Autodesk Inventor part; units mm, degrees
ref_plane "YZ Plane" through (0, 0, 0) normal (1, 0, 0) x (0, 1, 0)
ref_plane "XZ Plane" through (0, 0, 0) normal (0, 1, 0) x (-1, 0, 0)
ref_plane "XY Plane" through (0, 0, 0) normal (0, 0, 1) x (1, 0, 0)
sketch "Sketch1" plane through (0, 0, 0) normal (0, 1, 0) x (-1, 0, 0)
  circle A0 centre (0, 0) radius 15.875
  dimension "d0" = 31.75
extrude "Extrusion1" add sketch "Sketch1" along normal blind 2.4892
sketch "Sketch2" plane through (0, 2.4892, 0) normal (0, 1, 0) x (1, 0, 0)
  circle A0 centre (0, 0) radius 15.875
  circle A1 centre (0, 11.5062) radius 1.8542
  line L0 (0, 0) -> (0, 15.875)
  circle A2 centre (-9.9647, -5.7531) radius 1.8542
  circle A3 centre (9.9647, -5.7531) radius 1.8542
  circle A4 centre (0, -25.4) radius 15.875
  line L1 (0, 0) -> (0, -25.4)
  circle A5 centre (21.997, 12.7) radius 15.875
  circle A6 centre (-21.997, 12.7) radius 15.875
  dimension "d3" = 3.7084
  dimension "d4" = 11.5062
  dimension "d7" = 360
  dimension "d9" = 31.75
  dimension "d10" = 25.4
  dimension "d13" = 360
extrude "Extrusion2" cut sketch "Sketch2" against normal through all contours A0 A5 | A0 A5 | A4 A0 | A0 L1 A4 | A6 A0 | A0 A6 | A0 A4 L1
sketch "Sketch6" plane through (0, 2.4892, 0) normal (0, 1, 0) x (1, 0, 0)
  arc A0 (-15.761, -1.8989) -> (-9.525, -12.7) centre (0, 0) ccw
  arc A1 (6.236, 14.5989) -> (-6.236, 14.5989) centre (0, 0) ccw
  line L0 (0, 0) -> (0, 11.5062)
  circle A2 centre (0, 11.5062) radius 1.8542
  circle A3 centre (-9.9647, -5.7531) radius 1.8542
  circle A4 centre (9.9647, -5.7531) radius 1.8542
  arc A5 (9.525, -12.7) -> (15.761, -1.8989) centre (0, 0) ccw
  circle A6 centre (0, 0) radius 4.5
  dimension "d26" = 11.5062
  dimension "d27" = 3.7084
  dimension "d30" = 360
  dimension "d34" = 9
extrude "Extrusion5" cut sketch "Sketch6" against normal through all
sketch "Sketch3" plane through (0, 2.4892, 0) normal (0, 1, 0) x (1, 0, 0)
  arc A0 (9.525, -12.7) -> (15.761, -1.8989) centre (0, 0) ccw
  circle A1 centre (0, 0) radius 5.9944
  line L0 (0, -7.3323) -> (-6.35, 3.6662)
  line L1 (-6.35, 3.6662) -> (6.35, 3.6662)
  line L2 (6.35, 3.6662) -> (0, -7.3323)
  line L3 (0, 0) -> (0, -8.4562)
  dimension "d17" = 11.9888
  dimension "d18" = 12.7
extrude "Extrusion3" add sketch "Sketch3" along normal blind 10.0076
sketch "Sketch4" plane through (0, 12.4968, 0) normal (0, 1, 0) x (1, 0, 0)
  arc A0 (-5.5463, 2.2741) -> (-0.8037, -5.9403) centre (0, 0) ccw
  circle A1 centre (0, 0) radius 3.9687
  dimension "d21" = 7.9375
extrude "Extrusion4" cut sketch "Sketch4" against normal through all
thread "Thread1"
properties part number "5_16_18_tee_nut"
Verification items for the finished model (mm, model axes). A direction names the side the tool comes from. Round coordinates to 2 decimals unless told otherwise and drop trailing zeros. Order: outer loops, then holes, each group sorted by start corner. A loop starts at its lowest first (then second) coordinate and runs counter-clockwise, first axis right, second up.
1. Section check D-D on z = 3.25. Record the cut outline in (x, y).
Final values:
outline: (-15.54, 0) - (-3.11, 0) - (-3.11, 2.49) - (-2.28, 2.49) - (-2.28, 12.5) - (-5.04, 12.5) - (-5.04, 2.49) - (-15.54, 2.49) - close; (2.28, 2.49) - (3.11, 2.49) - (3.11, 0) - (15.54, 0) - (15.54, 2.49) - (5.04, 2.49) - (5.04, 12.5) - (2.28, 12.5) - close
2. Section check B-B on x = -10. Record the cut outline in (y, z), then the cut area to 3 significant figures.
Final values:
outline: (0, -2.3) - (2.49, -2.3) - (2.49, 3.9) - (0, 3.9) - close; (0, 7.61) - (2.49, 7.61) - (2.49, 12.33) - (0, 12.33) - close
area: 27.2 mm2
3. Go/stop test with flat-tipped pins: P1, Ø1.8, axis at x = 6, y = 7.5, coming from the -Z side; P2, Ø1.5, axis at x = 12.5, y = 1.5, coming from the +Z side; P3, Ø3, axis at y = 7, z = -0.5, coming from the +X side. Record where each tip stops, or that it passes through.
Final values:
P1: stops at z = -3.67
P2: stops at z = 10.67
P3: stops at x = 5.99
4. Access from +Z, -Z, +X, -X, +Y, -Y to the whole of each face (thin tool, end or side, straight path). Record for faces 5 (the flat face through (5.954, 7.423, -2.98)), 6 (the flat face through (-6, 7, -3.666)), 7 (the flat face through (6, 7, -3.666)), 8 (the cylindrical face through (-0.59, 1.26, -4.46)), 9 (the flat face through (-0.396, 7.423, 6.646)).
Final values:
face 5: +X, +Y
face 6: -Z, -X, +Y
face 7: -Z, +X, +Y
face 8: -Y
face 9: +Z, -X, +Y
5. Thickness scan on L1, parallel to Z at x = 0, y = 1.45 (3 decimals); L2, parallel to X at y = 5.25, z = 0; L3, parallel to Z at x = -0.5, y = 7. Record the ranges inside material, lowest first.
Final values:
L1: z = -15.875 to -13.36, -9.652 to -4.5, 4.5 to 9.525
L2: x = -5.99 to -3.97, 3.97 to 5.99
L3: z = -5.97 to -3.94, 3.94 to 6.47
6. Release check for a two-part mould opening along X. For faces 1 (the cylindrical face through (5.23, 7.42, 2.93)), 2 (the flat face through (0, 0, -5)), 3 (the cylindrical face through (-0.077, 7.423, -5.994)), 4 (the cylindrical face through (0.143, 1.262, 9.526)) record: +X half, -X half, draft (parallel to the pull), parting line (faces both ways), or undercut.
Final values:
face 1: +X half
face 2: draft
face 3: parting line
face 4: undercut
7. Section check A-A on y = 6.5. Record the cut outline in (x, z), then the cut area to 3 significant figures.
Final values:
outline: (-6.35, -3.67) - (-4.74, -3.67) arc R5.99 ccw to (4.74, -3.67) - (6.35, -3.67) - (5.55, -2.27) arc R5.99 ccw to (0.8, 5.94) - (0, 7.33) - (-0.8, 5.94) arc R5.99 ccw to (-5.55, -2.27) - close; hole circle Ø7.94 at (0, 0)
area: 66.6 mm2
8. Section check C-C on z = 0. Record the cut outline in (x, y).
Final values:
outline: (-12.47, 0) - (-4.5, 0) - (-4.5, 2.49) - (-3.97, 2.49) - (-3.97, 12.5) - (-5.99, 12.5) - (-5.99, 2.49) - (-12.47, 2.49) - close; (3.97, 2.49) - (4.5, 2.49) - (4.5, 0) - (12.47, 0) - (12.47, 2.49) - (5.99, 2.49) - (5.99, 12.5) - (3.97, 12.5) - close
